The figure shows three views and two pictorial views of one solid part (mm, origin at its lowest corner). Answer the questions. Round coordinates to 2 decimals unless told otherwise and drop trailing zeros. Order: outer loops, then holes, each group sorted by start corner. A loop starts at its lowest first (then second) coordinate and runs counter-clockwise, first axis right, second up. Notation, with made-up numbers: M 45.25,-23 L 85.25,-23 A22 ccw 85.25,16 Z; hole C 36,-31.5 d5. An arc over 180 degrees is marked long. Return JSON: item names as keys, results as strings.
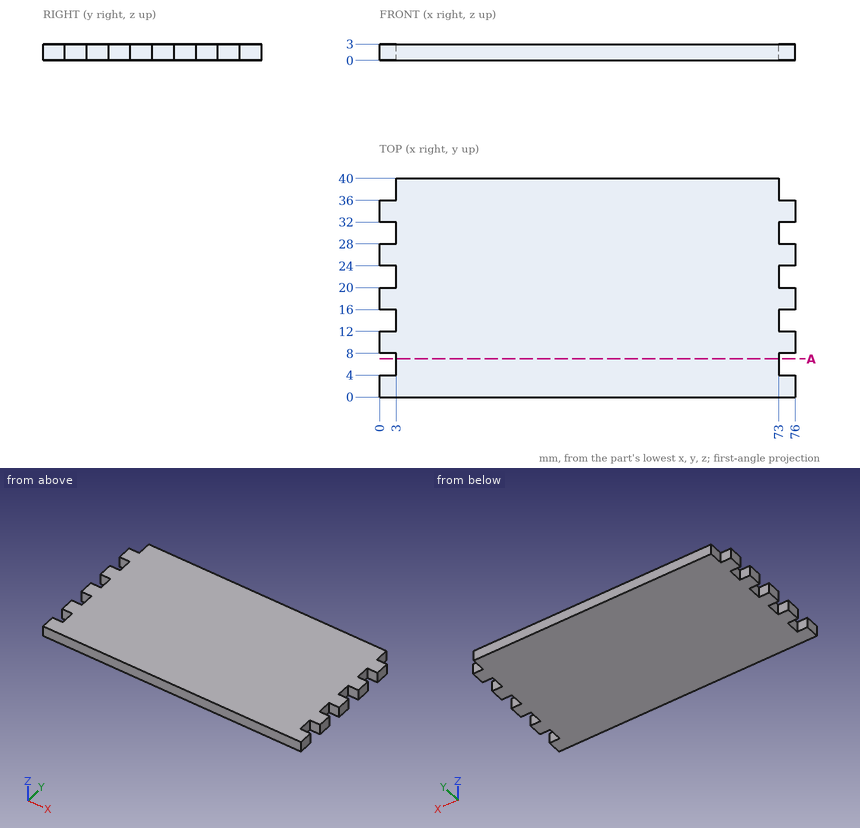
Item 1: Find section A-A (y = 7). Determine the outline of the cut face in (x, z), plus the area to 3 significant figures.
Output:
{"outline": "M 3,0 L 73,0 L 73,3 L 3,3 Z", "area": "210 mm^2"}
Item 2: Each of these flat-tipped pins is pushed along its axis until it touches: pin 1 (0.9 mm diameter, centred on x = 1.5, z = 2, fed in from +Y); pin 2 (1.5 mm diameter, centred on y = 37.5, z = 2, fed in from +X); pin 3 (0.9 mm diameter, centred on y = 31, z = 2, fed in from -X). Where does it stop, or does it pass through?
Output:
{"pin 1": "stops at y = 36", "pin 2": "stops at x = 73", "pin 3": "stops at x = 3"}
Item 3: Consider line 1 along X through (y, z) = (5.5, 2.85). Determine where the line is inside the solid, lowest interval first. Write a range as [from, to].
Output:
{"line 1": "x = [3, 73]"}
